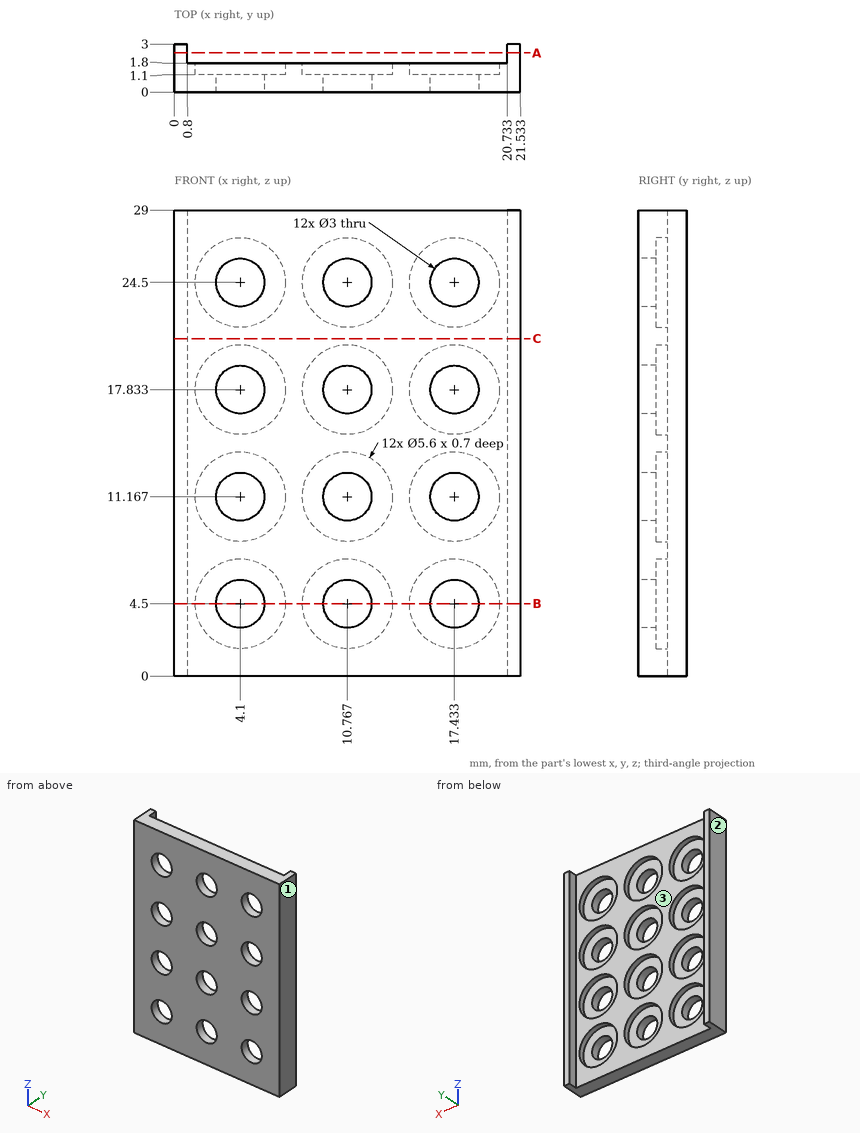
Print and shaded views of the part. All mm, measured from the part's lowest x, y and z. Coordinates: 2 decimals unless noted, no trailing zeros. Loops run counter-clockwise (first coordinate to the right, second up) from the corner with the lowest first, then second, coordinate; pieces in that order, holes last. Notation, with made-up numbers: (37.25, 30.25) -> (55.25, 30.25) arc R28 cw to (55.25, 67.25) -> close; hole circle Ø4 at (-5, 65). An arc over 180 degrees is marked (long way). Use a Markdown table: item, result. Add a question column.
Item 1: Flat gauge pins, fed straight in: P1, Ø4, axis at x = 4.1, z = 24.5, coming from the +Y side; P2, Ø4.5, axis at x = 4.5, z = 16.5, coming from the +Y side; P3, Ø2.5, axis at x = 17.43, z = 4.5, coming from the +Y side. Where does each tip first touch, or does it go through?
Item 2: Probe probe 1 along Z at (x, y) = (10.75, 0.9); probe 2 along X at (y, z) = (0.8, 24.5); probe 3 along X at (y, z) = (0.55, 12) (1 decimal). List the from-to ranges inside material, lowest first.
Item 3: Pull direction X, two halves, no side cores. Call the marked faces 1, 2 and 3: +X half, -X half, draft (parallel to the pull), parting line (faces both ways), or undercut.
Item 4: Band-saw the part on B-B on z = 4.5. Give the number of separate pieces and of enclosed holes in the cut face.
Item 5: Band-saw the part on A-A on y = 2.45. Write the cut outline in (x, z).
Item 6: Band-saw the part on C-C on z = 21. Write the cut outline in (x, y).
Geometry says:
| question | item | result |
|---|---|---|
| 1 | P1 | y = 1.1 |
| 1 | P2 | y = 1.8 |
| 1 | P3 | through |
| 2 | probe 1 | 0 to 3, 6 to 9.67, 12.67 to 16.33, 19.33 to 23, 26 to 29 |
| 2 | probe 2 | 0 to 2.6, 5.6 to 9.27, 12.27 to 15.93, 18.93 to 21.53 |
| 2 | probe 3 | 0 to 2.9, 5.3 to 9.5, 12 to 16.2, 18.7 to 21.5 |
| 3 | face 1 | +X half |
| 3 | face 2 | -X half |
| 3 | face 3 | undercut |
| 4 | separate pieces | 4 |
| 4 | enclosed holes | 0 |
| 5 | outline | (0, 0) -> (0.8, 0) -> (0.8, 29) -> (0, 29) -> close; (20.73, 0) -> (21.53, 0) -> (21.53, 29) -> (20.73, 29) -> close |
| 6 | outline | (0, 0) -> (21.53, 0) -> (21.53, 3) -> (20.73, 3) -> (20.73, 1.8) -> (0.8, 1.8) -> (0.8, 3) -> (0, 3) -> close |
